Autodesk Inventor part; units mm, degrees
ref_plane "YZ Plane" through (0, 0, 0) normal (1, 0, 0) x (0, 1, 0)
ref_plane "XZ Plane" through (0, 0, 0) normal (0, 1, 0) x (-1, 0, 0)
ref_plane "XY Plane" through (0, 0, 0) normal (0, 0, 1) x (1, 0, 0)
sketch "Sketch1" plane through (0, 0, 0) normal (0, 0, 1) x (1, 0, 0)
  point P0 (0, 0)
sketch "Sketch2" plane through (0, 0, 0) normal (0, 0, 1) x (1, 0, 0)
  line L0 (-100, -34.5) -> (-100, 34.5)
  circle A0 centre (-60, 22) radius 1.4998
  circle A1 centre (-60, -22) radius 1.4998
  circle A2 centre (-89.5, 25) radius 1.4998
  circle A3 centre (-89.5, -25) radius 1.4998
  circle A4 centre (-39.5, 25) radius 1.4998
  circle A5 centre (-39.5, -25) radius 1.4998
  circle A6 centre (-89.5, 25) radius 14.1598
  circle A7 centre (-89.5, -25) radius 14.1598
  line L1 (0, 34.5) -> (0, -34.5)
  line L2 (0, 34.5) -> (-100, 34.5)
  line L3 (0, -34.5) -> (-100, -34.5)
  point P0 (-100, 15.5)
  point P1 (-100, -15.5)
  point P2 (-79, -34.5)
  point P3 (-79, 34.5)
extrude "Extrusion1" add sketch "Sketch2" along normal blind 3
fillet "Fillet1" radius 5 2 edges at (0, 34.5, 1.5) (0, -34.5, 1.5)
properties part number "Power Distribution Board redo v2" material "CFRP"
Check sheet for the modelled part. Datum: model origin and axes. Units: mm. Round coordinates to 2 decimals unless told otherwise and drop trailing zeros. Loops run counter-clockwise (first coordinate to the right, second up) from the corner with the lowest first, then second, coordinate; pieces in that order, holes last.
1. Scan lines: probe 1 along Y at (x, z) = (-89.5, 1); probe 2 along Y at (x, z) = (-60, 0.85); probe 3 along X at (y, z) = (25.5, 1.5). Record each from-to range of solid material in increasing order.
2. Mould release check, pull along Y, two halves, no side actions. Record for faces 1 (the flat face through (-41, 34.5, 1)), 2 (the flat face through (-53, 1, 3)), 3 (the flat face through (-100, 0, 1)), 4 (the flat face through (-41, -34.5, 1)): released by +Y, released by -Y, zero draft, split by the parting line, or undercut.
3. Sectioned sample at B-B on x = -60. Record the boundary of the cut face in (y, z).
4. Sectioned sample at D-D on y = -22. Record the boundary of the cut face in (x, z), and give its area (3 significant figures).
5. Gauge pin test, flat ends, axial feed: pin 1 Ø5 at (x, y) = (-60, 22) entering from +Z; pin 2 Ø1 at (y, z) = (13.5, 1.5) entering from -X; pin 3 Ø1.5 at (x, z) = (-48, 0.5) entering from -Y; pin 4 Ø1.5 at (x, z) = (-37.5, 1.5) entering from +Y. Record the tip position at first contact, or that the pin passes through.
6. Sectioned sample at C-C on z = 0.55. Record the boundary of the cut face in (x, y), and give its area (3 significant figures).
7. Sectioned sample at A-A on y = 25. Record the boundary of the cut face in (x, z).
Recorded:
1. probe 1: y = -39.16 to -26.5, -23.5 to 23.5, 26.5 to 39.16
1. probe 2: y = -34.5 to -23.5, -20.5 to 20.5, 23.5 to 34.5
1. probe 3: x = -103.65 to -90.91, -88.09 to -40.91, -38.09 to 0
2. face 1: released by +Y
2. face 2: zero draft
2. face 3: undercut
2. face 4: released by -Y
3. outline: (-34.5, 0) - (-23.5, 0) - (-23.5, 3) - (-34.5, 3) - close; (-20.5, 0) - (20.5, 0) - (20.5, 3) - (-20.5, 3) - close; (23.5, 0) - (34.5, 0) - (34.5, 3) - (23.5, 3) - close
4. outline: (-103.34, 0) - (-61.5, 0) - (-61.5, 3) - (-103.34, 3) - close; (-58.5, 0) - (0, 0) - (0, 3) - (-58.5, 3) - close
4. area: 301 mm2
5. pin 1: stops at z = 3
5. pin 2: stops at x = -100
5. pin 3: stops at y = -34.5
5. pin 4: stops at y = 34.5
6. outline: (-100, -15.5) arc R14.16 ccw to (-79, -34.5) - (-5, -34.5) arc R5 ccw to (0, -29.5) - (0, 29.5) arc R5 ccw to (-5, 34.5) - (-79, 34.5) arc R14.16 ccw to (-100, 15.5) - close; hole circle Ø3 at (-89.5, -25); hole circle Ø3 at (-89.5, 25); hole circle Ø3 at (-60, -22); hole circle Ø3 at (-60, 22); hole circle Ø3 at (-39.5, -25); hole circle Ø3 at (-39.5, 25)
6. area: 7,080 mm2
7. outline: (-103.66, 0) - (-91, 0) - (-91, 3) - (-103.66, 3) - close; (-88, 0) - (-41, 0) - (-41, 3) - (-88, 3) - close; (-38, 0) - (0, 0) - (0, 3) - (-38, 3) - close
